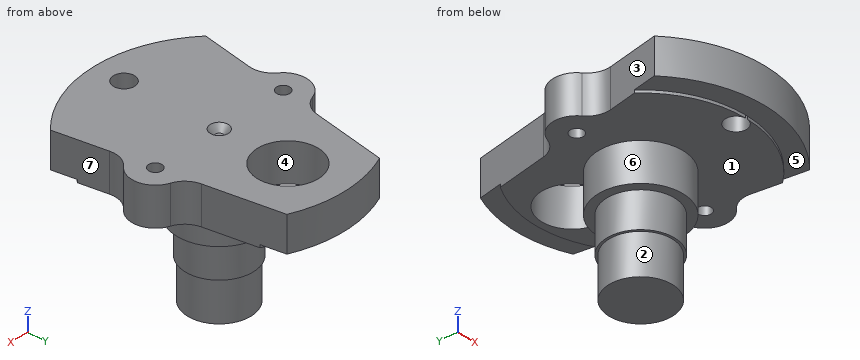
```python
from build123d import *

# Parameters (mm, degrees)
SKETCH1_R           = 3.090826528
SKETCH1_R_2         = 14.35
SKETCH1_R_3         = 5
BOSS_EXTRUDE1_DEPTH = 18
SKETCH2_R           = 20
BOSS_EXTRUDE2_DEPTH = 18
SKETCH3_R           = 16
BOSS_EXTRUDE3_DEPTH = 35.7
SKETCH5_OUTSIDE_W   = 123.14
SKETCH5_OUTSIDE_H   = 152.554
SKETCH5_OUTSIDE_R   = 14.935
CUT_EXTRUDE1_DEPTH  = 19
SKETCH6_R           = 14.35
CUT_EXTRUDE2_DEPTH  = 22.35
SKETCH7_R           = 4.25
CUT_EXTRUDE3_DEPTH  = 3
CUT_EXTRUDE3_DRAFT  = -38
SKETCH9_OUTSIDE_W   = 123.14
SKETCH9_OUTSIDE_H   = 152.554
SKETCH9_OUTSIDE_R   = 49.923055682
CUT_EXTRUDE4_DEPTH  = 1.35


with BuildPart() as part:
    # Sketch1 → Boss-Extrude1 (new body)
    with BuildSketch(Plane.XY):
        with BuildLine():
            Line((36.136520686, -18.774478422), (40.195752281, -43.049171521))
            ThreePointArc((40.195752281, -43.049171521), (0, -58.897620241), (-40.195752281, -43.049171521))
            Line((-40.195752281, -43.049171521), (-36.136520686, -18.774478422))
            ThreePointArc((-36.136520686, -18.774478422), (-36.697665198, -13.197066935), (-40.010085223, -8.674868838))
            ThreePointArc((-40.010085223, -8.674868838), (-44.039037615, 1.827589449), (-36.814887741, 10.449987378))
            ThreePointArc((-36.814887741, 10.449987378), (-32.208677837, 13.651878045), (-29.862109135, 18.747257211))
            Line((-29.862109135, 18.747257211), (-24.003146652, 53.784557457))
            ThreePointArc((-24.003146652, 53.784557457), (0, 58.897620241), (24.003146652, 53.784557457))
            Line((24.003146652, 53.784557457), (29.862109135, 18.747257211))
            ThreePointArc((29.862109135, 18.747257211), (32.208677837, 13.651878045), (36.814887741, 10.449987378))
            ThreePointArc((36.814887741, 10.449987378), (44.039037615, 1.827589449), (40.010085223, -8.674868838))
            ThreePointArc((40.010085223, -8.674868838), (36.697665198, -13.197066935), (36.136520686, -18.774478422))
        make_face()
        with Locations((-33.1, 0)):
            Circle(SKETCH1_R, mode=Mode.SUBTRACT)
        with Locations(Location((33.1, 0, 0), (0, 0, 180))):
            Circle(SKETCH1_R, mode=Mode.SUBTRACT)
        with Locations((0, 32.4)):
            Circle(SKETCH1_R_2, mode=Mode.SUBTRACT)
        with Locations((0.004379967, -44.949999787)):
            Circle(SKETCH1_R_3, mode=Mode.SUBTRACT)
    extrude(amount=-BOSS_EXTRUDE1_DEPTH)

    # Sketch2 → Boss-Extrude2 (add)
    with BuildSketch(Plane(origin=(0, 0, -18), x_dir=(-1, 0, 0), z_dir=(0, 0, -1))):
        with Locations(Location((0, 0, 0), (0, 0, 106.311047481))):
            Circle(SKETCH2_R)
    extrude(amount=BOSS_EXTRUDE2_DEPTH)

    # Sketch3 → Boss-Extrude3 (add)
    with BuildSketch(Plane(origin=(0, 0, -36), x_dir=(-1, 0, 0), z_dir=(0, 0, -1))):
        with Locations(Location((0, 0, 0), (0, 0, 180))):
            Circle(SKETCH3_R)
    extrude(amount=BOSS_EXTRUDE3_DEPTH)

    # Sketch5 outside → Cut-Extrude1 (cut)
    with BuildSketch(Plane(origin=(0, 0, -71.7), x_dir=(-1, 0, 0), z_dir=(0, 0, -1))):
        Rectangle(SKETCH5_OUTSIDE_W, SKETCH5_OUTSIDE_H)
        Circle(SKETCH5_OUTSIDE_R, mode=Mode.SUBTRACT)
    extrude(amount=-CUT_EXTRUDE1_DEPTH, mode=Mode.SUBTRACT)

    # Sketch6 → Cut-Extrude2 (cut)
    with BuildSketch(Plane.XY):
        with Locations((0, 32.4)):
            Circle(SKETCH6_R)
    extrude(amount=-CUT_EXTRUDE2_DEPTH, mode=Mode.SUBTRACT)


with BuildPart() as cut_extrude3_tool:
    # Sketch7 → Cut-Extrude3 (with draft: the straight prism first)
    with BuildSketch(Plane.XY):
        Circle(SKETCH7_R)
    extrude(amount=-CUT_EXTRUDE3_DEPTH)
    # Cut-Extrude3: the draft: its side faces are tilted about the plane it starts from
    cut_extrude3_sides = [cut_extrude3_tool.faces().sort_by_distance(p)[0] for p in [
        (-4.25, 0, -1.5),
    ]]
    draft(cut_extrude3_sides, Plane.XY, CUT_EXTRUDE3_DRAFT)


with BuildPart() as part_1:
    add(part.part)

    # Cut-Extrude3: cut by cut_extrude3_tool
    add(cut_extrude3_tool.part, mode=Mode.SUBTRACT)

    # Sketch9 outside → Cut-Extrude4 (cut)
    with BuildSketch(Plane(origin=(0, 0, -18), x_dir=(-1, 0, 0), z_dir=(0, 0, -1))):
        Rectangle(SKETCH9_OUTSIDE_W, SKETCH9_OUTSIDE_H)
        Circle(SKETCH9_OUTSIDE_R, mode=Mode.SUBTRACT)
    extrude(amount=-CUT_EXTRUDE4_DEPTH, mode=Mode.SUBTRACT)


solid = part_1.part
```
The model under review builds one solid part; all positions refer to its coordinate system, in mm. Face numbers are marked on the shaded views. A direction names the side the tool comes from. Round coordinates to 2 decimals unless told otherwise and drop trailing zeros. Order: outer loops, then holes, each group sorted by start corner. A loop starts at its lowest first (then second) coordinate and runs counter-clockwise, first axis right, second up. Notation, with made-up numbers: (50, 38) -> (89, 38) arc R34 ccw to (89, 75) -> close; hole circle Ø11 at (50.25, 30.5). An arc over 180 degrees is marked (long way). Use a Markdown table: item, result.
Q1. Clearance check with flat-ended pins moving along their axes: P1, Ø3.5, axis at x = 33.1, y = 0, coming from the +Z side; P2, Ø1.5, axis at y = -1, z = -53.5, coming from the +X side; P3, Ø1, axis at x = 2.5, y = 18.5, coming from the +Z side; P4, Ø13.5, axis at x = -17, y = -44, coming from the -Z side. State where each tip first meets the part, or that it passes through.
Values:
| item | result |
|---|---|
| P1 | passes through |
| P2 | stops at x = 14.93 |
| P3 | stops at z = 0 |
| P4 | stops at z = -18 |
Q2. We need section D-D on x = 33.1. Write out the cut boundary in (y, z).
Values:
| item | result |
|---|---|
| outline | (-48.72, -16.65) -> (-37.37, -16.65) -> (-37.37, -18) -> (-3.09, -18) -> (-3.09, 0) -> (-48.72, 0) -> close; (3.09, -18) -> (12.71, -18) -> (12.71, 0) -> (3.09, 0) -> close |
Q3. Tool access review of the marked faces 4, 5, 6 and 7: name each direction out of +Z, -Z, +X, -X, +Y, -Y from which nothing blocks a thin tool from reaching the whole face with its end or side.
Values:
| item | result |
|---|---|
| face 4 | +Z |
| face 5 | -Z, -Y |
| face 6 | -Z |
| face 7 | +Z, -Z, +X |
Q4. Mouldability with a two-part tool opening along Y and no side actions: class the marked faces 1, 2 and 3 as +Y half, -Y half, draft (parallel to the pull), parting line (faces both ways), or undercut.
Values:
| item | result |
|---|---|
| face 1 | draft |
| face 2 | parting line |
| face 3 | undercut |
Q5. We need section C-C on y = -44.95. Write out the cut boundary in (x, z).
Values:
| item | result |
|---|---|
| outline | (-38.06, -16.65) -> (-21.72, -16.65) -> (-21.72, -18) -> (-5, -18) -> (-5, 0) -> (-38.06, 0) -> close; (5, -18) -> (21.72, -18) -> (21.72, -16.65) -> (38.06, -16.65) -> (38.06, 0) -> (5, 0) -> close |
Q6. We need section A-A on y = 0. Write out the cut boundary in (x, z) (3 decimals), then the cut area to 3 significant figures.
Values:
| item | result |
|---|---|
| outline | (-44.191, -18) -> (-36.191, -18) -> (-36.191, 0) -> (-44.191, 0) -> close; (-30.009, -18) -> (-20, -18) -> (-20, -36) -> (-16, -36) -> (-16, -52.7) -> (-14.935, -52.7) -> (-14.935, -71.7) -> (14.935, -71.7) -> (14.935, -52.7) -> (16, -52.7) -> (16, -36) -> (20, -36) -> (20, -18) -> (30.009, -18) -> (30.009, 0) -> (4.25, 0) -> (1.906, -3) -> (-1.906, -3) -> (-4.25, 0) -> (-30.009, 0) -> close; (36.191, -18) -> (44.191, -18) -> (44.191, 0) -> (36.191, 0) -> close |
| area | 3,170 mm^2 |
Q7. For line 1 (Y direction, x = 0, z = -7.25); line 2 (Y direction, x = 0, z = -17.5); line 3 (Z direction, x = -13, y = -37.5), list the stretches that pass through material, from the lowest coordinate up.
Values:
| item | result |
|---|---|
| line 1 | y = -58.9 to -49.95, -39.95 to 18.05, 46.75 to 58.9 |
| line 2 | y = -39.95 to 18.05, 46.75 to 49.92 |
| line 3 | z = -18 to 0 |
Q8. We need section B-B on z = -13.5. Write out the cut boundary in (x, y), then the cut area to 3 significant figures.
Values:
| item | result |
|---|---|
| outline | (-40.2, -43.05) arc R58.9 ccw to (40.2, -43.05) -> (36.14, -18.77) arc R10.66 cw to (40.01, -8.67) arc R11.09 ccw to (36.81, 10.45) arc R10.67 cw to (29.86, 18.75) -> (24, 53.78) arc R58.9 ccw to (-24, 53.78) -> (-29.86, 18.75) arc R10.67 cw to (-36.81, 10.45) arc R11.09 ccw to (-40.01, -8.67) arc R10.66 cw to (-36.14, -18.77) -> close; hole circle Ø6.18 at (-33.1, 0); hole circle Ø28.7 at (0, 32.4); hole circle Ø10 at (0, -44.95); hole circle Ø6.18 at (33.1, 0) |
| area | 6,900 mm^2 |
